Part model, mm, in its own coordinate system. Face numbers are marked on the shaded views. A direction names the side the tool comes from. Give positions to 0.01 mm unless a question says otherwise; leave off trailing zeros. Loops run counter-clockwise (first coordinate to the right, second up) from the corner with the lowest first, then second, coordinate; pieces in that order, holes last. Notation, with made-up numbers: (42.5, -3) -> (46.5, -3) arc R12 cw to (46.5, 10) -> close; hole circle Ø10 at (49, 4). An arc over 180 degrees is marked (long way). One line per question, with ' | ' between items.
```python
from build123d import *

# Parameters (mm, degrees)
SKETCH1_W           = 40
SKETCH1_H           = 24.2
SKETCH1_H_2         = 5.8
BOSS_EXTRUDE1_DEPTH = 10
SKETCH2_W           = 26.88873999
SKETCH2_H           = 5
BOSS_EXTRUDE2_DEPTH = 100
SKETCH3_R           = 1.5
CUT_EXTRUDE1_DEPTH  = 30
SKETCH6_W           = 8
SKETCH6_H           = 25
BOSS_EXTRUDE3_DEPTH = 10
CUT_EXTRUDE4_DEPTH  = 35
BOSS_EXTRUDE4_DEPTH = 10
SKETCH9_W           = 8
SKETCH9_H           = 15
BOSS_EXTRUDE5_DEPTH = 30
CUT_EXTRUDE5_DEPTH  = 35
SKETCH11_R          = 1.42
CUT_EXTRUDE6_DEPTH  = 20
SKETCH12_R          = 3
CUT_EXTRUDE7_DEPTH  = 3
FILLET1_R           = 10
CHAMFER1_SIZE       = 1
CHAMFER2_SIZE       = 1


with BuildPart() as part:
    # Sketch1 → Boss-Extrude1 (new body)
    with BuildSketch(Plane(origin=(0, 0, 0), x_dir=(1, 0, 0), z_dir=(0, 1, 0))):
        with Locations((0, -2.9)):
            Rectangle(SKETCH1_W, SKETCH1_H)
        with Locations((0, 12.1)):
            Rectangle(SKETCH1_W, SKETCH1_H_2)
    extrude(amount=BOSS_EXTRUDE1_DEPTH)

    # Sketch2 → Boss-Extrude2 (add)
    with BuildSketch(Plane(origin=(0, 10, 0), x_dir=(1, 0, 0), z_dir=(0, 1, 0))):
        with Locations((6.555630005, 12.5)):
            Rectangle(SKETCH2_W, SKETCH2_H)
    extrude(amount=BOSS_EXTRUDE2_DEPTH)

    # Sketch3 → Cut-Extrude1 (cut)
    with BuildSketch(Plane.XY.offset(-10)):
        with Locations((9, 96.14)):
            Circle(SKETCH3_R)
    extrude(amount=-CUT_EXTRUDE1_DEPTH, mode=Mode.SUBTRACT)

    # Sketch6 → Boss-Extrude3 (add)
    with BuildSketch(Plane(origin=(0, 10, 0), x_dir=(1, 0, 0), z_dir=(0, 1, 0))):
        with Locations((0, -2.5)):
            Rectangle(SKETCH6_W, SKETCH6_H)
    extrude(amount=BOSS_EXTRUDE3_DEPTH)

    # Sketch7 → Cut-Extrude4 (cut)
    with BuildSketch(Plane.ZY.offset(4)):
        Polygon((-10, 21.535084573), (15, 10), (15, 21.535084573), align=None)
    extrude(amount=-CUT_EXTRUDE4_DEPTH, mode=Mode.SUBTRACT)

    # Sketch8 → Boss-Extrude4 (add)
    with BuildSketch(Plane(origin=(0, 0, 0), x_dir=(1, 0, 0), z_dir=(0, 1, 0))):
        Polygon((-20, 30), (-20, 15), (20, 15), (20, 23.768276438), (4, 23.768276438), (4, 30), align=None)
    extrude(amount=BOSS_EXTRUDE4_DEPTH)

    # Sketch9 → Boss-Extrude5 (add)
    with BuildSketch(Plane(origin=(0, 10, 0), x_dir=(1, 0, 0), z_dir=(0, 1, 0))):
        with Locations((0, 22.5)):
            Rectangle(SKETCH9_W, SKETCH9_H)
    extrude(amount=BOSS_EXTRUDE5_DEPTH)

    # Sketch10 → Cut-Extrude5 (cut)
    with BuildSketch(Plane.ZY.offset(4)):
        Polygon((-30, 10), (-20.186840819, 40), (-30, 40), align=None)
    extrude(amount=-CUT_EXTRUDE5_DEPTH, mode=Mode.SUBTRACT)

    # Sketch11 → Cut-Extrude6 (cut)
    with BuildSketch(Plane(origin=(0, 10, 0), x_dir=(1, 0, 0), z_dir=(0, 1, 0))):
        with Locations(Location((-12, -7, 0), (0, 0, 270))):
            Circle(SKETCH11_R)
        with Locations(Location((12, -7, 0), (0, 0, 270))):
            Circle(SKETCH11_R)
        with Locations(Location((-12, 23, 0), (0, 0, 270))):
            Circle(SKETCH11_R)
    extrude(amount=-CUT_EXTRUDE6_DEPTH, mode=Mode.SUBTRACT)

    # Sketch12 → Cut-Extrude7 (cut)
    with BuildSketch(Plane(origin=(0, 10, 0), x_dir=(1, 0, 0), z_dir=(0, 1, 0))):
        with Locations(Location((-12, -7, 0), (0, 0, 270))):
            Circle(SKETCH12_R)
        with Locations(Location((12, -7, 0), (0, 0, 270))):
            Circle(SKETCH12_R)
        with Locations(Location((-12, 23, 0), (0, 0, 270))):
            Circle(SKETCH12_R)
    extrude(amount=-CUT_EXTRUDE7_DEPTH, mode=Mode.SUBTRACT)

    # Fillet1
    fillet1_edges = [part.edges().sort_by_distance(p)[0] for p in [
        (-6.88873999, 110, -12.5),
        (20, 110, -12.5),
    ]]
    fillet(fillet1_edges, radius=FILLET1_R)

    # Chamfer1
    chamfer1_edges = [part.edges().sort_by_distance(p)[0] for p in [
        (4, 25, -25.093420409),
        (-4, 25, -25.093420409),
    ]]
    chamfer(chamfer1_edges, length=CHAMFER1_SIZE)

    # Chamfer2
    chamfer2_edges = [part.edges().sort_by_distance(p)[0] for p in [
        (4, 15, 4.163495143),
    ]]
    chamfer(chamfer2_edges, length=CHAMFER2_SIZE)


solid = part.part
```
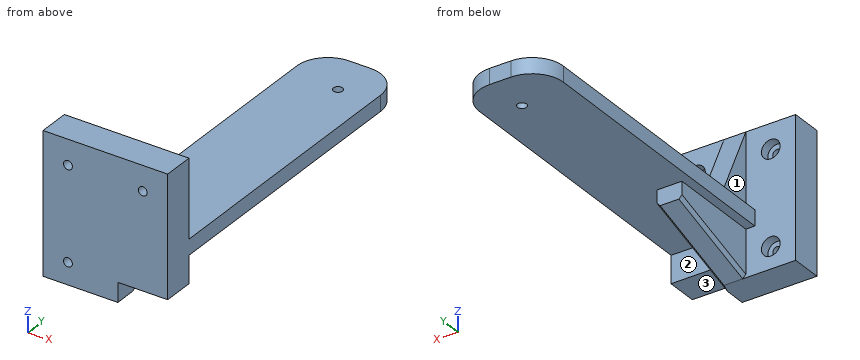
1) Saw through at B-B (z = -11.5). Give the cut face in (x, y), and give its area (3 significant figures).
Found:
outline: (-20, 0) -> (20, 0) -> (20, 100) arc R10 ccw to (10, 110) -> (3.11, 110) arc R10 ccw to (-6.89, 100) -> (-6.89, 10) -> (-20, 10) -> close; hole circle Ø3 at (9, 96.14) | area: 3,040 mm2
2) Pin check, flat tips, straight feed: P1, Ø4, axis at y = 29.5, z = -18.5, coming from the -X side; P2, Ø3, axis at x = 9, y = 4, coming from the -Z side; P3, Ø2.5, axis at x = -12, z = -23, coming from the +Y side; P4, Ø5, axis at x = 15.5, z = 8, coming from the +Y side. Stop position of each tip, or through.
Found:
P1: x = -4 | P2: z = -23.77 | P3: through | P4: y = 10
3) Saw through at C-C (x = 6). Give the cut face in (y, z), and give its area (3 significant figures).
Found:
outline: (0, -23.77) -> (10, -23.77) -> (10, -15) -> (110, -15) -> (110, -10) -> (10, -10) -> (10, 15) -> (0, 15) -> close | area: 888 mm2
4) Drill centre lines: line 1 (X direction, y = 8, z = 7); line 2 (X direction, y = 4, z = -23); line 3 (Y direction, x = 9.5, z = -3.5). Where is each one in solid material? Low to high.
Found:
line 1: -20 to -15, -9 to 9, 15 to 20 | line 2: -20 to -13.42, -10.58 to 20 | line 3: 0 to 10
5) Tool access for the marked faces 1, 2 and 3: list every direction of +Z, -Z, +X, -X, +Y, -Y with a clear straight run to the whole face (end or side of a thin tool).
Found:
face 1: +Z, -X, +Y | face 2: -Z, +X, +Y | face 3: -Z, +X, +Y, -Y
6) Saw through at A-A (x = -12). Give the cut face in (y, z).
Found:
outline: (0, -30) -> (10, -30) -> (10, -26) -> (7, -26) -> (7, -24.42) -> (0, -24.42) -> close; (0, -21.58) -> (7, -21.58) -> (7, -20) -> (10, -20) -> (10, 4) -> (7, 4) -> (7, 5.58) -> (0, 5.58) -> close; (0, 8.42) -> (7, 8.42) -> (7, 10) -> (10, 10) -> (10, 15) -> (0, 15) -> close
7) Saw through at D-D (y = 16). Give the cut face in (x, z), and give its area (3 significant figures).
Found:
outline: (-6.89, -15) -> (-4, -15) -> (-4, -26.99) -> (-3, -28.04) -> (3, -28.04) -> (4, -26.99) -> (4, -15) -> (20, -15) -> (20, -10) -> (4, -10) -> (4, -0.39) -> (3, 2) -> (-4, 2) -> (-4, -10) -> (-6.89, -10) -> close | area: 332 mm2
